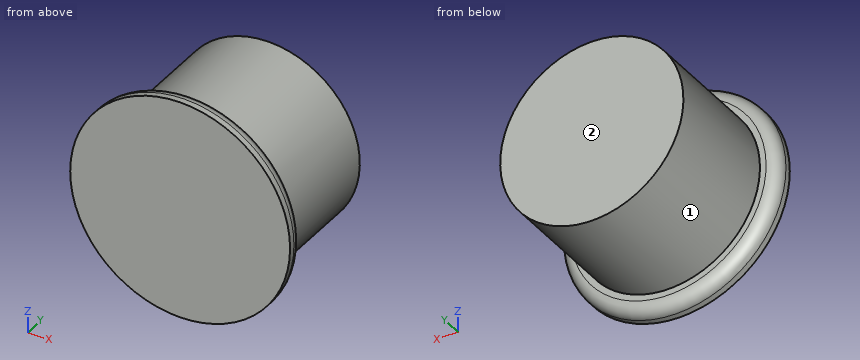
```python
from build123d import *

# Parameters (mm, degrees)
ESBO_O1_R                = 9
RESSALTO_EXTRUS_O1_DEPTH = 1.5
FILETE1_R                = 1
ESBO_O2_R                = 7.5
RESSALTO_EXTRUS_O2_DEPTH = 10


with BuildPart() as part:
    # Esboço1 → Ressalto-extrusão1 (new body)
    with BuildSketch(Plane(origin=(0, 0, 0), x_dir=(1, 0, 0), z_dir=(0, 1, 0))):
        with Locations(Location((0, 0, 0), (0, 0, 270))):
            Circle(ESBO_O1_R)
    extrude(amount=RESSALTO_EXTRUS_O1_DEPTH)

    # Filete1
    filete1_edges = [part.edges().sort_by_distance(p)[0] for p in [
        (0, 1.5, -9),
    ]]
    fillet(filete1_edges, radius=FILETE1_R)

    # Esboço2 → Ressalto-extrusão2 (add)
    with BuildSketch(Plane(origin=(0, 1.5, 0), x_dir=(1, 0, 0), z_dir=(0, 1, 0))):
        with Locations(Location((0, 0, 0), (0, 0, 270))):
            Circle(ESBO_O2_R)
    extrude(amount=RESSALTO_EXTRUS_O2_DEPTH)


solid = part.part
```
Input: part model. Units: mm. Frame: model coordinates. Face numbers are marked on the shaded views. A direction names the side the tool comes from. Round coordinates to 2 decimals unless told otherwise and drop trailing zeros. Order: outer loops, then holes, each group sorted by start corner. A loop starts at its lowest first (then second) coordinate and runs counter-clockwise, first axis right, second up. Notation, with made-up numbers: (49.25, 71) - (60.25, 71) arc R9 ccw to (60.25, 83) - close; hole circle Ø11 at (66, 32.25). An arc over 180 degrees is marked (long way). Answer in a Markdown table with one row per item.
Item 1: Line query: line 1 (Y direction, x = -2.5, z = -7.5); line 2 (Z direction, x = 6.75, y = 8.25); line 3 (Z direction, x = -6, y = 4). Output: solid intervals per line, ascending.
Model answer:
| item | result |
|---|---|
| line 1 | y = 0 to 1.5 |
| line 2 | z = -3.27 to 3.27 |
| line 3 | z = -4.5 to 4.5 |
Item 2: Section query A-A (z = 0). Return the cut outline in (x, y), then the cut area to 3 significant figures.
Model answer:
| item | result |
|---|---|
| outline | (-9, 0) - (9, 0) - (9, 0.5) arc R1 ccw to (8, 1.5) - (7.5, 1.5) - (7.5, 11.5) - (-7.5, 11.5) - (-7.5, 1.5) - (-8, 1.5) arc R1 ccw to (-9, 0.5) - close |
| area | 177 mm² |
Item 3: Pin query (flat end, axial travel): pin 1 (3 mm diameter, centred on x = 2.5, y = 10, fed in from -Z); pin 2 (3 mm diameter, centred on y = 9, z = 0.5, fed in from -X); pin 3 (5 mm diameter, centred on x = -6, y = 3.5, fed in from -Z); pin 4 (4 mm diameter, centred on y = 2, z = 1.5, fed in from +X). Return the tip coordinate at first contact, or that it passes through.
Model answer:
| item | result |
|---|---|
| pin 1 | stops at z = -7.43 |
| pin 2 | stops at x = -7.5 |
| pin 3 | stops at z = -7.14 |
| pin 4 | stops at x = 9 |
Item 4: Reachability of the marked faces 1 and 2 from +Z, -Z, +X, -X, +Y, -Y: full face, straight path, thin tool, end or side. Return the list, or none.
Model answer:
| item | result |
|---|---|
| face 1 | +Y |
| face 2 | +Z, -Z, +X, -X, +Y |
Item 5: Section query B-B (y = 4). Return the cut outline in (x, z), then the cut area to 3 significant figures.
Model answer:
| item | result |
|---|---|
| outline | circle Ø15 at (0, 0) |
| area | 177 mm² |
